from build123d import *

# Parameters (mm, degrees)
F1_DEPTH       = 28
F2_W           = 30
F2_H           = 30
F3_DEPTH       = 4
F5_D           = 3.3
F5_DEPTH       = 40
F5_CSINK_D     = 6.72
F5_CSINK_ANGLE = 90
F5_TIP         = 0.9914200214
F7_D           = 3.3
F7_DEPTH       = 40
F7_CSINK_D     = 6.72
F7_CSINK_ANGLE = 90
F7_TIP         = 0.9914200214
F9_D           = 3.3
F9_DEPTH       = 40
F9_CSINK_D     = 6.72
F9_CSINK_ANGLE = 90
F9_TIP         = 0.9914200214


with BuildPart() as f1:
    # F0 (on Front) → F1 (new body)
    with BuildSketch(Plane.XZ):
        Polygon((0, 4), (0, 0), (4, 0), (30, 0), (30, 4), (4, 4), (4, 30), (0, 30), align=None)
    extrude(amount=F1_DEPTH)

    # F2 (on face) → F3 (join)
    with BuildSketch(Plane.XZ.offset(28)):
        with Locations((15, 15)):
            Rectangle(F2_W, F2_H)
    extrude(amount=F3_DEPTH)

    # F5
    with Locations(Plane.XZ.offset(32)):
        with Locations((15, 15)):
            CounterSinkHole(F5_D / 2, F5_CSINK_D / 2, depth=F5_DEPTH, counter_sink_angle=F5_CSINK_ANGLE)
            with Locations((0, 0, -(F5_DEPTH + F5_TIP / 2))):  # 118° drill point
                Cone(0, F5_D / 2, F5_TIP, mode=Mode.SUBTRACT)

    # F7
    with Locations(Plane(origin=(0, 0, 0), x_dir=(0, -1, 0), z_dir=(-1, 0, 0))):
        with Locations((16, 15)):
            CounterSinkHole(F7_D / 2, F7_CSINK_D / 2, depth=F7_DEPTH, counter_sink_angle=F7_CSINK_ANGLE)
            with Locations((0, 0, -(F7_DEPTH + F7_TIP / 2))):  # 118° drill point
                Cone(0, F7_D / 2, F7_TIP, mode=Mode.SUBTRACT)

    # F9
    with Locations(Plane(origin=(0, 0, 0), x_dir=(1, 0, 0), z_dir=(0, 0, -1))):
        with Locations((15, 16)):
            CounterSinkHole(F9_D / 2, F9_CSINK_D / 2, depth=F9_DEPTH, counter_sink_angle=F9_CSINK_ANGLE)
            with Locations((0, 0, -(F9_DEPTH + F9_TIP / 2))):  # 118° drill point
                Cone(0, F9_D / 2, F9_TIP, mode=Mode.SUBTRACT)


solid = f1.part
The model under review builds one solid part; all positions refer to its coordinate system, in mm. A direction names the side the tool comes from. Give positions to 0.01 mm unless a question says otherwise; leave off trailing zeros. Loops run counter-clockwise (first coordinate to the right, second up) from the corner with the lowest first, then second, coordinate; pieces in that order, holes last. Notation, with made-up numbers: (33, 20.5) -> (45, 20.5) arc R14 cw to (45, 25.5) -> close; hole circle Ø11 at (-28.75, -21.5). An arc over 180 degrees is marked (long way). Put each result on its own line as item: value. Start each with the question number.
1. Clearance check with flat-ended pins moving along their axes: P1, Ø2, axis at x = 15, z = 15, coming from the +Y side; P2, Ø2, axis at x = 7.5, y = -16, coming from the +Z side; P3, Ø13, axis at y = -11.5, z = 19, coming from the +X side; P4, Ø8, axis at x = 15, z = 17, coming from the +Y side. State where each tip first meets the part, or that it passes through.
2. Mouldability with a two-part tool opening along Z and no side actions: class faces 1 (the face through (4, -14, 17)), 2 (the face through (13.476, -29.129, 14.368)), 3 (the face through (3.8, -20.7, 30)), 4 (the face through (2.871, -14.476, 14.368)) as released by +Z, released by -Z, zero draft, split by the parting line, or undercut.
3. We need section A-A on x = 15. State the section outline as (y, z) points, then the cut area to 3 significant figures.
4. We need section B-B on z = 15. State the section outline as (x, y) points.
5. For faces 5 (the face through (17, -28, 17)), 6 (the face through (11, -16, 0)), list the 3-axis set-ups (+Z, -Z, +X, -X, +Y, -Y) from which the entire face can be reached by the end or side of a thin tool; tool diameter is ignored.
6. We need section C-C on y = -6.5. State the section outline as (x, z) points.
7. Wall thickness on probe 1 along Y at (x, z) = (15, 3.5); probe 2 along X at (y, z) = (-16, 3.1): over which ranges is each line inside the solid? List them lowest first.
8. We need section D-D on x = 23.5. State the section outline as (y, z) points.
Determined:
1. P1: through
1. P2: z = 4
1. P3: x = 4
1. P4: y = -28
2. face 1: zero draft
2. face 2: undercut
2. face 3: released by +Z
2. face 4: undercut
3. outline: (-32, 0) -> (-19.36, 0) -> (-17.65, 1.71) -> (-17.65, 4) -> (-28, 4) -> (-28, 13.35) -> (-30.29, 13.35) -> (-32, 11.64) -> close; (-32, 18.36) -> (-30.29, 16.65) -> (-28, 16.65) -> (-28, 30) -> (-32, 30) -> close; (-14.35, 1.71) -> (-12.64, 0) -> (0, 0) -> (0, 4) -> (-14.35, 4) -> close
3. area: 200 mm^2
4. outline: (0, -32) -> (11.64, -32) -> (13.35, -30.29) -> (13.35, -28) -> (4, -28) -> (4, -17.65) -> (1.71, -17.65) -> (0, -19.36) -> close; (0, -12.64) -> (1.71, -14.35) -> (4, -14.35) -> (4, 0) -> (0, 0) -> close; (16.65, -30.29) -> (18.36, -32) -> (30, -32) -> (30, -28) -> (16.65, -28) -> close
5. face 5: +Z, +X, +Y
5. face 6: -Z, +X, -X, +Y, -Y
6. outline: (0, 0) -> (30, 0) -> (30, 4) -> (4, 4) -> (4, 30) -> (0, 30) -> close
7. probe 1: -32 to -17.65, -14.35 to 0
7. probe 2: 0 to 13.35, 16.65 to 30
8. outline: (-32, 0) -> (0, 0) -> (0, 4) -> (-28, 4) -> (-28, 30) -> (-32, 30) -> close
